Geometry: final body of the model. Coordinates: model frame, mm. A direction names the side the tool comes from. Round coordinates to 2 decimals unless told otherwise and drop trailing zeros. Loops run counter-clockwise (first coordinate to the right, second up) from the corner with the lowest first, then second, coordinate; pieces in that order, holes last. Notation, with made-up numbers: (-25, -5.5) - (20, -5.5) arc R20 cw to (20, 7.5) - close; hole circle Ø7 at (65.5, 66). An arc over 180 degrees is marked (long way). Return JSON: item names as keys, results as strings. Group by question number.
1. Material intervals for probe 1 along Y at (x, z) = (-44.5, -6); probe 2 along Z at (x, y) = (-1, 71); probe 3 along Z at (x, y) = (-10, 80.5), sorted ascending.
2. Set-up query: faces 1 (the face through (23, 0, -23)), 2 (the face through (0, 100, 0)). Return all of +Z, -Z, +X, -X, +Y, -Y with unobstructed straight access to the full face (end or side cutting, diameter ignored); none if empty.
3. Section A-A on z = 0. Return loops of the section in (x, y).
4. Section D-D on y = -7.5. Return loops of the section in (x, z).
5. Section C-C on y = 63. Return loops of the section in (x, z).
6. First-contact query: pin 1 Ø8 at (y, z) = (83, 28.5) entering from -X; pin 2 Ø12 at (x, y) = (-6, 62.5) entering from -Z; pin 3 Ø10 at (x, y) = (-27.5, 47) entering from -Z. Flat tips, straight axial feed; report the tip coordinate or a pass-through.
7. Section B-B on x = 0. Return loops of the section in (y, z).
from build123d import *

# Parameters (mm, degrees)
F0_R     = 54
F0_R_2   = 30
F1_DEPTH = 20
F2_DEPTH = 100
F3_SIZE  = 0.5


with BuildPart() as f1:
    # F0 (on Front) → F1 (new body)
    with BuildSketch(Plane.XZ):
        Circle(F0_R)
        Circle(F0_R_2, mode=Mode.SUBTRACT)
        Circle(F0_R_2)
    extrude(amount=F1_DEPTH)

    # F0 (on Front) → F2 (join)
    with BuildSketch(Plane.XZ):
        Circle(F0_R_2)
    extrude(amount=-F2_DEPTH)

    # F3
    f3_edges = [f1.edges().sort_by_distance(p)[0] for p in [
        (-54, -20, 0),
        (54, -10, 0),
        (-54, 0, 0),
        (-30, 100, 0),
    ]]
    chamfer(f3_edges, length=F3_SIZE)


solid = f1.part
Taken from the geometry:
{
 "1": {"probe 1": "-20 to 0", "probe 2": "-29.98 to 29.98", "probe 3": "-28.28 to 28.28"},
 "2": {"face 1": "+Y", "face 2": "+Z, -Z, +X, -X, +Y"},
 "3": {"outline": "(-54, -19.5) - (-53.5, -20) - (53.5, -20) - (54, -19.5) - (54, -0.5) - (53.5, 0) - (30, 0) - (30, 99.5) - (29.5, 100) - (-29.5, 100) - (-30, 99.5) - (-30, 0) - (-53.5, 0) - (-54, -0.5) - close"},
 "4": {"outline": "circle Ø108 at (0, 0)"},
 "5": {"outline": "circle Ø60 at (0, 0)"},
 "6": {"pin 1": "x = -17.31", "pin 2": "z = -30", "pin 3": "z = -19.84"},
 "7": {"outline": "(-20, -53.5) - (-19.5, -54) - (-0.5, -54) - (0, -53.5) - (0, -30) - (99.5, -30) - (100, -29.5) - (100, 29.5) - (99.5, 30) - (0, 30) - (0, 53.5) - (-0.5, 54) - (-19.5, 54) - (-20, 53.5) - close"}
}
